The listing builds one solid part. Answer for the finished solid, in the listing's coordinates (mm). A direction names the side the tool comes from. Coordinates: 2 decimals unless noted, no trailing zeros. Order: outer loops, then holes, each group sorted by start corner. A loop starts at its lowest first (then second) coordinate and runs counter-clockwise, first axis right, second up. Notation, with made-up numbers: (5.5, 14) -> (54.5, 14) arc R23 cw to (54.5, 34) -> close; hole circle Ø5 at (69, 71). An arc over 180 degrees is marked (long way). Return JSON: item names as keys, results as strings.
from build123d import *

# Parameters (mm, degrees)
SKETCH_1_R                      = 3
EXTRUDE_1_DEPTH                 = 1
EXTRUDE_2_DEPTH                 = 1
EXTRUDE_2_DEPTH_BACK            = 1
FILLET_1_R                      = 1
SKETCH_3_R                      = 2
EXTRUDE_3_DEPTH                 = 8.4
EXTRUDE_4_DEPTH                 = 2
CHAMFER_1_SIZE                  = 0.5
CHAMFER_2_SIZE                  = 1
CUT_EXTRUDE_1_REACH             = 11.775
CUT_EXTRUDE_1_DIRECTION_2_REACH = 11.775


with BuildPart() as part:
    # 草图1 → 凸台-拉伸1 (new body)
    with BuildSketch(Plane(origin=(0, 0, 0), x_dir=(1, 0, 0), z_dir=(0, 1, 0))):
        with Locations(Location((0, 0, 0), (0, 0, 270))):
            Circle(SKETCH_1_R)
    extrude(amount=EXTRUDE_1_DEPTH)

    # 草图2 → 凸台-拉伸2 (add, two sides: drawn at the far end of the back side and taken through both)
    with BuildSketch(Plane.XY.offset(-EXTRUDE_2_DEPTH_BACK)):
        Polygon((-3.75, 7), (3.75, 7), (4, 1), (-4, 1), align=None)
    extrude(amount=EXTRUDE_2_DEPTH + EXTRUDE_2_DEPTH_BACK)

    # 圆角1
    fillet_1_edges = [part.edges().sort_by_distance(p)[0] for p in [
        (-3.75, 7, 0),
        (3.75, 7, 0),
    ]]
    fillet(fillet_1_edges, radius=FILLET_1_R)

    # 草图3 → 凸台-拉伸3 (add)
    with BuildSketch(Plane(origin=(0, 0, 0), x_dir=(-1, 0, 0), z_dir=(0, -1, 0))):
        with Locations(Location((0, 0, 0), (0, 0, 270))):
            Circle(SKETCH_3_R)
    extrude(amount=EXTRUDE_3_DEPTH)

    # 草图4 → 凸台-拉伸4 (add)
    with BuildSketch(Plane(origin=(0, -8.4, 0), x_dir=(-1, 0, 0), z_dir=(0, -1, 0))):
        with BuildLine():
            Line((2.598076211, -1.5), (-2.598076211, -1.5))
            ThreePointArc((-2.598076211, -1.5), (-3, 0), (-2.598076211, 1.5))
            Line((-2.598076211, 1.5), (2.598076211, 1.5))
            ThreePointArc((2.598076211, 1.5), (3, 0), (2.598076211, -1.5))
        make_face()
    extrude(amount=-EXTRUDE_4_DEPTH)

    # 倒角1
    chamfer_1_edges = [part.edges().sort_by_distance(p)[0] for p in [
        (3, -8.4, 0),
        (-3, -8.4, 0),
    ]]
    chamfer(chamfer_1_edges, length=CHAMFER_1_SIZE)

    # 倒角2
    chamfer_2_edges = [part.edges().sort_by_distance(p)[0] for p in [
        (3, -6.4, 0),
        (-3, -6.4, 0),
    ]]
    chamfer(chamfer_2_edges, length=CHAMFER_2_SIZE - 0.0001)  # a hair under: the kernel refuses the full size

    # 草图5 → 切除-拉伸1 (cut, up to next)
    with BuildSketch(Plane(origin=(0, 0, 0), x_dir=(0, 0, -1), z_dir=(1, 0, 0)), mode=Mode.PRIVATE) as cut_extrude_1_sk1:
        Polygon((2, -5.2), (1, -8.4), (2, -8.4), align=None)
    cut_extrude_1_tool1 = extrude(cut_extrude_1_sk1.sketch, amount=-CUT_EXTRUDE_1_REACH, mode=Mode.PRIVATE) & part.part
    # 草图5 → 切除-拉伸1 (cut, up to next)
    with BuildSketch(Plane(origin=(0, 0, 0), x_dir=(0, 0, -1), z_dir=(1, 0, 0)), mode=Mode.PRIVATE) as cut_extrude_1_sk2:
        Polygon((-2, -5.2), (-2, -8.4), (-1, -8.4), align=None)
    cut_extrude_1_tool2 = extrude(cut_extrude_1_sk2.sketch, amount=-CUT_EXTRUDE_1_REACH, mode=Mode.PRIVATE) & part.part
    add(cut_extrude_1_tool1.solids().sort_by_distance((0, -7.333333, -1.666667))[0], mode=Mode.SUBTRACT)
    add(cut_extrude_1_tool2.solids().sort_by_distance((0, -7.333333, 1.666667))[0], mode=Mode.SUBTRACT)

    # 草图5 → 切除-拉伸1 direction 2 (cut, up to next)
    with BuildSketch(Plane(origin=(0, 0, 0), x_dir=(0, 0, -1), z_dir=(1, 0, 0)), mode=Mode.PRIVATE) as cut_extrude_1_direction_2_sk1:
        Polygon((2, -5.2), (1, -8.4), (2, -8.4), align=None)
    cut_extrude_1_direction_2_tool1 = extrude(cut_extrude_1_direction_2_sk1.sketch, amount=CUT_EXTRUDE_1_DIRECTION_2_REACH, mode=Mode.PRIVATE) & part.part
    # 草图5 → 切除-拉伸1 direction 2 (cut, up to next)
    with BuildSketch(Plane(origin=(0, 0, 0), x_dir=(0, 0, -1), z_dir=(1, 0, 0)), mode=Mode.PRIVATE) as cut_extrude_1_direction_2_sk2:
        Polygon((-2, -5.2), (-2, -8.4), (-1, -8.4), align=None)
    cut_extrude_1_direction_2_tool2 = extrude(cut_extrude_1_direction_2_sk2.sketch, amount=CUT_EXTRUDE_1_DIRECTION_2_REACH, mode=Mode.PRIVATE) & part.part
    add(cut_extrude_1_direction_2_tool1.solids().sort_by_distance((0, -7.333333, -1.666667))[0], mode=Mode.SUBTRACT)
    add(cut_extrude_1_direction_2_tool2.solids().sort_by_distance((0, -7.333333, 1.666667))[0], mode=Mode.SUBTRACT)


solid = part.part
1. Each of these flat-tipped pins is pushed along its axis until it touches: pin 1 Ø1 at (x, z) = (-1, -2.5) entering from +Y; pin 2 Ø1.8 at (x, y) = (1.5, 3.5) entering from -Z; pin 3 Ø2 at (y, z) = (-1.5, 2) entering from -X. Where does it stop, or does it pass through?
Answer block:
{"pin 1": "stops at y = 1", "pin 2": "stops at z = -1", "pin 3": "stops at x = -1.73"}
2. For faces 5 (the face through (0, 4, -1)), 6 (the face through (0.9, 0.49, 2.86)), 7 (the face through (0, 1, 2)), determine the directions among +Z, -Z, +X, -X, +Y, -Y from which every point of the face is accessible in a straight line to the end or side of a thin tool.
Answer block:
{"face 5": "-Z, +X, -X, +Y", "face 6": "-Y", "face 7": "+Z, +X, -X, +Y"}
3. Consider line 1 (Z direction, x = 1, y = 2.25); line 2 (X direction, y = -3.25, z = 1.5); line 3 (Y direction, x = -2.25, z = 0.6). Determine where each line is inside the solid, lowest interval first. Write a range as from..to.
Answer block:
{"line 1": "z = -1..1", "line 2": "x = -1.32..1.32", "line 3": "y = -8.4..-6.73, 0..7"}
4. The part is cut by section C-C on y = -5.75. Give the vertices of the cut face in (x, z), and give its area (3 significant figures).
Answer block:
{"outline": "(-0.81, -1.83) -> (0.81, -1.83) arc R2 ccw to (0.81, 1.83) -> (-0.81, 1.83) arc R2 ccw to start", "area": "12.2 mm2"}
5. Determine the mould class of faces 1 (the face through (1.2, -3.4, -1.6)), 2 (the face through (0, 7, 0)), 3 (the face through (0, 4, 1)), 4 (the face through (2.4, -6.8, 0)) for opening direction Y: pulls with the +Y half, pulls with the -Y half, needs draft (parallel to the pull), parting line crosses it, or undercut.
Answer block:
{"face 1": "undercut", "face 2": "pulls with the +Y half", "face 3": "needs draft", "face 4": "undercut"}
6. The part is cut by section B-B on z = -1.8. Give the vertices of the cut face in (x, y).
Answer block:
{"outline": "(-2.4, 0) -> (-0.87, 0) -> (-0.87, -5.84) -> (0.87, -5.84) -> (0.87, 0) -> (2.4, 0) -> (2.4, 1) -> (-2.4, 1) -> close"}
7. The part is cut by section D-D on y = 1.5. Give the vertices of the cut face in (x, z), and give its area (3 significant figures).
Answer block:
{"outline": "(-3.98, -1) -> (3.98, -1) -> (3.98, 1) -> (-3.98, 1) -> close", "area": "15.9 mm2"}
8. The part is cut by section A-A on x = 0. Give the vertices of the cut face in (y, z), and give its area (3 significant figures).
Answer block:
{"outline": "(-8.4, -1) -> (-5.2, -2) -> (0, -2) -> (0, -3) -> (1, -3) -> (1, -1) -> (7, -1) -> (7, 1) -> (1, 1) -> (1, 3) -> (0, 3) -> (0, 2) -> (-5.2, 2) -> (-8.4, 1) -> close", "area": "48.4 mm2"}
